Work out the finished part from the listing and answer in its coordinate system (mm). A direction names the side the tool comes from. Give positions to 0.01 mm unless a question says otherwise; leave off trailing zeros. Order: outer loops, then holes, each group sorted by start corner. A loop starts at its lowest first (then second) coordinate and runs counter-clockwise, first axis right, second up. Notation, with made-up numbers: (65.25, 17) - (88.25, 17) arc R28 cw to (88.25, 53) - close; hole circle Ø6 at (-1, -32.75). An arc over 180 degrees is marked (long way). Put each result on its own line as item: value.
```python
from build123d import *

# Parameters (mm, degrees)
SKETCH1_W             = 50
SKETCH1_H             = 16.5
BOSS_EXTRUDE1_DEPTH   = 6.5
LPATTERN1_COUNT       = 2
LPATTERN1_PITCH       = 20
SKETCH4_R             = 3.25
CUT_EXTRUDE1_DEPTH    = 51
M3X0_5_TAPPED_HOLE2_D = 2.5
LPATTERN2_COUNT       = 2
LPATTERN2_PITCH       = 20
LPATTERN2_COUNT_DIR2  = 2
LPATTERN2_PITCH_DIR2  = 5
SKETCH9_W             = 17
SKETCH9_H             = 1
BOSS_EXTRUDE2_DEPTH   = 2


with BuildPart() as part:
    # Sketch1 → Boss-Extrude1 (new body, symmetric)
    with BuildSketch(Plane.XY):
        Rectangle(SKETCH1_W, SKETCH1_H)
    extrude(amount=BOSS_EXTRUDE1_DEPTH, both=True)

    # Sketch2 → M3x0.5 Tapped Hole1 (revolve, cut)
    with BuildSketch(Plane(origin=(10, 8.25, 0), x_dir=(0, 0, 1), z_dir=(1, 0, 0))):
        Polygon((0, 0), (0, 7.5), (1.25, 6.748924226), (1.25, 0), align=None)
    m3x0_5_tapped_hole1 = revolve(axis=Axis((10, 14.6, 0), (0, -1, 0)), mode=Mode.SUBTRACT)

    # LPattern1: M3x0.5 Tapped Hole1 ×2
    with Locations(*[(-i * LPATTERN1_PITCH, 0, 0) for i in range(1, LPATTERN1_COUNT)]):
        add(m3x0_5_tapped_hole1, mode=Mode.SUBTRACT)

    # Sketch4 → Cut-Extrude1 (cut, through all)
    with BuildSketch(Plane(origin=(25, 0, 0), x_dir=(0, 0, -1), z_dir=(1, 0, 0))):
        with Locations((0, 0.75)):
            Circle(SKETCH4_R)
    extrude(amount=-CUT_EXTRUDE1_DEPTH, mode=Mode.SUBTRACT)

    # M3x0.5 Tapped Hole2 (through all)
    with Locations(Plane(origin=(25, 0, 0), x_dir=(0, 0, -1), z_dir=(1, 0, 0))):
        with Locations((0, -4.25)):
            Hole(M3X0_5_TAPPED_HOLE2_D / 2)

    # Sketch7 → M3x0.5 Tapped Hole3 (revolve, cut)
    with BuildSketch(Plane(origin=(-10, 0.75, 6.5), x_dir=(0, -1, 0), z_dir=(1, 0, 0))):
        Polygon((0, 0), (0, 7.5), (1.25, 6.748924226), (1.25, 0), align=None)
    m3x0_5_tapped_hole3 = revolve(axis=Axis((-10, 0.75, 12.85), (0, 0, -1)), mode=Mode.SUBTRACT)

    # LPattern2: M3x0.5 Tapped Hole3 2 × 2
    with Locations(*[(i * LPATTERN2_PITCH, -j * LPATTERN2_PITCH_DIR2, 0) for i in range(LPATTERN2_COUNT) for j in range(LPATTERN2_COUNT_DIR2) if (i, j) != (0, 0)]):
        add(m3x0_5_tapped_hole3, mode=Mode.SUBTRACT)

    # Sketch9 → Boss-Extrude2 (add)
    with BuildSketch(Plane.XZ.offset(8.25)):
        with Locations((0, 4)):
            Rectangle(SKETCH9_W, SKETCH9_H)
    extrude(amount=BOSS_EXTRUDE2_DEPTH)


solid = part.part
```
(1) Determine the mould class of faces 5 (the face through (8.946, 6.031, 0.672)), 6 (the face through (0, 0, -6.5)), 7 (the face through (8.5, -9, 4)) for opening direction X: pulls with the +X half, pulls with the -X half, needs draft (parallel to the pull), parting line crosses it, or undercut.
Geometry check:
face 5: undercut
face 6: needs draft
face 7: pulls with the +X half
(2) Given pin 1 (2 mm diameter, centred on x = -2.5, y = -9.5, fed in from +Z); pin 2 (0.5 mm diameter, centred on y = -9, z = 4, fed in from +X); pin 3 (4 mm diameter, centred on x = 10, z = 0, fed in from -Y), each flat-ended and moving along its own axis, determine where each tip first touches the part or whether it passes through.
Geometry check:
pin 1: stops at z = 4.5
pin 2: stops at x = 8.5
pin 3: stops at y = -8.25
(3) Section A-A, the plane y = -4.25 is taken. Write down the section's boundary in (x, z).
Geometry check:
outline: (-25, -6.5) - (25, -6.5) - (25, -1.25) - (-25, -1.25) - close; (-25, 1.25) - (-11.25, 1.25) - (-11.25, 6.5) - (-25, 6.5) - close; (-8.75, 1.25) - (8.75, 1.25) - (8.75, 6.5) - (-8.75, 6.5) - close; (11.25, 1.25) - (25, 1.25) - (25, 6.5) - (11.25, 6.5) - close
(4) Section D-D, the plane y = 3.25 is taken. Write down the section's boundary in (x, z), then the cut area to 3 significant figures.
Geometry check:
outline: (-25, -6.5) - (25, -6.5) - (25, -2.08) - (-25, -2.08) - close; (-25, 2.08) - (25, 2.08) - (25, 6.5) - (-25, 6.5) - close
area: 442 mm²
(5) Section B-B, the plane z = 5.75 is taken. Write down the section's boundary in (x, y), then the cut area to 3 significant figures.
Geometry check:
outline: (-25, -8.25) - (25, -8.25) - (25, 8.25) - (-25, 8.25) - close; hole circle Ø2.5 at (-10, -4.25); hole circle Ø2.5 at (-10, 0.75); hole circle Ø2.5 at (10, -4.25); hole circle Ø2.5 at (10, 0.75)
area: 805 mm²
(6) Section C-C, the plane x = -4 is taken. Write down the section's boundary in (y, z), then the cut area to 3 significant figures.
Geometry check:
outline: (-10.25, 3.5) - (-8.25, 3.5) - (-8.25, -6.5) - (8.25, -6.5) - (8.25, 6.5) - (-8.25, 6.5) - (-8.25, 4.5) - (-10.25, 4.5) - close; hole circle Ø2.5 at (-4.25, 0); hole circle Ø6.5 at (0.75, 0)
area: 178 mm²
(7) Straight lines are drawn through the part: line 1 (X direction, y = 0.75, z = 4.4); line 2 (Y direction, x = 14, z = -0.25); line 3 (Y direction, x = 10, z = 4). For each, find the intervals that lie inside material, in ascending order.
Geometry check:
line 1: x = -25 to -11.25, -8.75 to 8.75, 11.25 to 25
line 2: y = -8.25 to -5.47, -3.03 to -2.49, 3.99 to 8.25
line 3: y = -8.25 to -5.5, -3 to -0.5, 2 to 8.25
(8) A tool of negligible diameter and unlimited length cuts with its end or side. For faces 1 (the face through (-11.24, 6.03, -0.16)), 2 (the face through (9.62, -0.44, 4.77)), 3 (the face through (0, -9, 3.5)), 4 (the face through (0, -9, 4.5)), from which of +Z, -Z, +X, -X, +Y, -Y can it reach the whole face along a straight path? Write none if from no direction.
Geometry check:
face 1: +Y
face 2: +Z
face 3: -Z, +X, -X, -Y
face 4: +Z, +X, -X, -Y
